```python
from build123d import *

# Parameters (mm, degrees)
BOSS_EXTRUDE1_DEPTH         = 7.9375
SKETCH2_R                   = 35.71875
BOSS_EXTRUDE2_DEPTH         = 1.5875
SKETCH3_R                   = 35.71875
CUT_EXTRUDE1_DEPTH          = 2.5875
CUT_EXTRUDE1_DEPTH_BACK     = 8.9375
F_6_CLEARANCE_HOLE1_D       = 4.3053
CUT_EXTRUDE2_DEPTH          = 6.604
F_0_257_DIAMETER_HOLE1_D    = 6.5278
F_51_0_067_DIAMETER_HOLE1_D = 1.7018


with BuildPart() as part:
    # Sketch1 → Boss-Extrude1 (new body)
    with BuildSketch(Plane.XY):
        with BuildLine():
            Line((-213.995000001, 2363.840725166), (-213.995000001, 2440.040725166))
            ThreePointArc((-213.995000001, 2440.040725166), (-214.92493597, 2442.285789196), (-217.170000001, 2443.215725166))
            Line((-217.170000001, 2443.215725166), (-293.370000001, 2443.215725166))
            ThreePointArc((-293.370000001, 2443.215725166), (-295.615064031, 2442.285789196), (-296.545000001, 2440.040725166))
            Line((-296.545000001, 2440.040725166), (-296.545000001, 2363.840725166))
            ThreePointArc((-296.545000001, 2363.840725166), (-295.615064031, 2361.595661136), (-293.370000001, 2360.665725166))
            Line((-293.370000001, 2360.665725166), (-217.170000001, 2360.665725166))
            ThreePointArc((-217.170000001, 2360.665725166), (-214.92493597, 2361.595661136), (-213.995000001, 2363.840725166))
        make_face()
    extrude(amount=-BOSS_EXTRUDE1_DEPTH)

    # Sketch2 → Boss-Extrude2 (add)
    with BuildSketch(Plane(origin=(0, 0, -7.9375), x_dir=(-1, 0, 0), z_dir=(0, 0, -1))):
        Polygon((282.257500001, 2360.665725166), (296.545000001, 2374.953225166), (296.545000001, 2428.928225166), (282.257500001, 2443.215725166), (228.282500001, 2443.215725166), (213.995000001, 2428.928225166), (213.995000001, 2374.953225166), (228.282500001, 2360.665725166), align=None)
        with Locations((255.270000001, 2401.940725166)):
            Circle(SKETCH2_R, mode=Mode.SUBTRACT)
    extrude(amount=BOSS_EXTRUDE2_DEPTH)

    # Sketch3 → Cut-Extrude1 (cut, two sides)
    with BuildSketch(Plane(origin=(0, 0, -7.9375), x_dir=(-1, 0, 0), z_dir=(0, 0, -1))) as cut_extrude1_sk:
        with Locations((255.270000001, 2401.940725166)):
            Circle(SKETCH3_R)
    extrude(amount=CUT_EXTRUDE1_DEPTH, mode=Mode.SUBTRACT)
    extrude(cut_extrude1_sk.sketch, amount=-CUT_EXTRUDE1_DEPTH_BACK, mode=Mode.SUBTRACT)

    # #6 Clearance Hole1 (through all)
    with Locations(Plane(origin=(0, 0, -7.9375), x_dir=(-1, 0, 0), z_dir=(0, 0, -1))):
        with Locations((217.170000001, 2440.040725166), (293.370000001, 2440.040725166), (293.370000001, 2363.840725166), (217.170000001, 2363.840725166)):
            Hole(F_6_CLEARANCE_HOLE1_D / 2)

    # Sketch6 → Cut-Extrude2 (cut)
    with BuildSketch(Plane.XY):
        with BuildLine():
            Line((-286.09833069, 2364.073109679), (-291.98898869, 2367.047457577))
            ThreePointArc((-291.98898869, 2367.047457577), (-293.256935443, 2368.521082635), (-293.111498919, 2370.459666654))
            Line((-293.111498919, 2370.459666654), (-290.083878389, 2376.455830423))
            ThreePointArc((-290.083878389, 2376.455830423), (-288.610253331, 2377.723777176), (-286.671669312, 2377.578340652))
            Line((-286.671669312, 2377.578340652), (-280.781011311, 2374.603992755))
            ThreePointArc((-280.781011311, 2374.603992755), (-279.513064558, 2373.130367697), (-279.658501082, 2371.191783678))
            Line((-279.658501082, 2371.191783678), (-282.686121613, 2365.195619909))
            ThreePointArc((-282.686121613, 2365.195619909), (-284.159746671, 2363.927673155), (-286.09833069, 2364.073109679))
        make_face()
    extrude(amount=-CUT_EXTRUDE2_DEPTH, mode=Mode.SUBTRACT)

    # F (0.257) Diameter Hole1 (through all)
    with Locations(Plane(origin=(0, 0, -9.525), x_dir=(-1, 0, 0), z_dir=(0, 0, -1))):
        with Locations((286.385000001, 2370.825725166)):
            Hole(F_0_257_DIAMETER_HOLE1_D / 2)

    # #51 (0.067) Diameter Hole1 (through all)
    with Locations(Plane(origin=(0, 0, -9.525), x_dir=(-1, 0, 0), z_dir=(0, 0, -1))):
        with Locations((290.619894526, 2373.004503404)):
            Hole(F_51_0_067_DIAMETER_HOLE1_D / 2)


solid = part.part
```
Work out the finished part from the listing and answer in its coordinate system (mm). A direction names the side the tool comes from. Round coordinates to 2 decimals unless told otherwise and drop trailing zeros. Write each loop counter-clockwise with the first axis right and the second up, starting at its lowest first coordinate (ties: lowest second). Pieces come first, ordered by that corner, then holes. Notation, with made-up numbers: (16, 27) -> (55, 27) arc R22 cw to (55, 53) -> close; hole circle Ø11 at (-10, -17). An arc over 180 degrees is marked (long way). Write each question's results on one line, items separated by ' | '.
1) The part is cut by section D-D (y = 2391). Write down the section's boundary in (x, z) (3 decimals), and give its area (3 significant figures).
Findings:
outline: (-296.545, -9.525) -> (-289.272, -9.525) -> (-289.272, 0) -> (-296.545, 0) -> close; (-221.268, -9.525) -> (-213.995, -9.525) -> (-213.995, 0) -> (-221.268, 0) -> close | area: 139 mm²
2) The part is cut by section A-A (x = -255.27). Write down the section's boundary in (y, z) (3 decimals).
Findings:
outline: (2360.666, -9.525) -> (2366.222, -9.525) -> (2366.222, 0) -> (2360.666, 0) -> close; (2437.659, -9.525) -> (2443.216, -9.525) -> (2443.216, 0) -> (2437.659, 0) -> close
3) Which of the six approach directions +Z, -Z, +X, -X, +Y, -Y give full straight-line access (tool end or side, diameter ignored) to faces 5 (the flat face through (-283.768, 2376.112, -3.256)), 6 (the flat face through (-221.04, 2367.91, -8.72)), 7 (the flat face through (-221.239, 2436.172, -8.72)), 8 (the flat face through (-289.501, 2435.972, -8.72))?
Findings:
face 5: +Z | face 6: -Z, +X, -Y | face 7: -Z, +X, +Y | face 8: -Z, -X, +Y
4) For a pull along X with two mould halves and no side action, classify faces 1 (the cylindrical face through (-292.38, 2438.13, -3.91)), 2 (the cylindrical face through (-214.9, 2442.26, -3.91)), 3 (the flat face through (-255, 2443.216, -5)), 4 (the cylindrical face through (-293.65, 2365.975, -3.913)) as +X half, -X half, draft (parallel to the pull), parting line (faces both ways), or undercut.
Findings:
face 1: undercut | face 2: +X half | face 3: draft | face 4: undercut
5) Flat-ended cylindrical pins translate along their axes: pin 1 (1.4 mm diameter, centred on x = -290.62, y = 2373, fed in from -Z); pin 2 (5.5 mm diameter, centred on x = -293.37, y = 2440.04, fed in from -Z); pin 3 (7 mm diameter, centred on x = -285.5, y = 2372.5, fed in from +Z). Find the tip coordinate at first contact, or state that the pin passes through.
Findings:
pin 1: passes through | pin 2: stops at z = -7.94 | pin 3: stops at z = -6.6
6) The part is cut by section C-C (z = -3). State how many separate pieces and enclosed holes the cut face has, and give its area (3 significant figures).
Findings:
separate pieces: 1 | enclosed holes: 6 | area: 2,610 mm²
7) Consider line 1 along X through (y, z) = (2439, -6.5) (3 decimals); line 2 along Y through (x, z) = (-263.5, -1.25); line 3 along X through (y, z) = (2378.5, -5.75) (3 decimals). Determine where each line is inside the solid, lowest interval first. Write a range as [from, to].
Findings:
line 1: x = [-296.545, -295.254], [-291.486, -219.054], [-215.286, -213.995] | line 2: y = [2360.67, 2367.18], [2436.7, 2443.22] | line 3: x = [-296.545, -282.221], [-228.319, -213.995]
8) The part is cut by section B-B (y = 2430). Write down the section's boundary in (x, z) (1 decimal).
Findings:
outline: (-296.5, -7.9) -> (-295.5, -7.9) -> (-295.5, -9.5) -> (-277.4, -9.5) -> (-277.4, 0) -> (-296.5, 0) -> close; (-233.2, -9.5) -> (-215.1, -9.5) -> (-215.1, -7.9) -> (-214, -7.9) -> (-214, 0) -> (-233.2, 0) -> close
